Build history of the part. All positions in model axes, mm. Face numbers are marked on the shaded views. A direction names the side the tool comes from. Round coordinates to 2 decimals unless told otherwise and drop trailing zeros. Write each loop counter-clockwise with the first axis right and the second up, starting at its lowest first coordinate (ties: lowest second). Pieces come first, ordered by that corner, then holes. Notation, with made-up numbers: (60, 11.5) -> (96, 11.5) arc R22 cw to (96, 22.5) -> close; hole circle Ø10 at (4, 26). An arc over 180 degrees is marked (long way). Return JSON: item names as keys, results as strings.
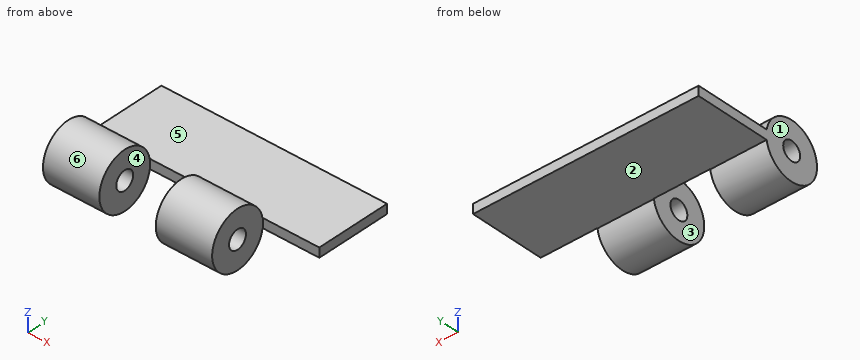
from build123d import *

# Parameters (mm, degrees)
F1_DEPTH = 1.5875
F2_W     = 19.05
F2_H     = 6.35


with BuildPart() as f1:
    # F0 (on Top) → F1 (new body, symmetric)
    with BuildSketch(Plane.XY):
        Polygon((76.2, 31.75), (0, 31.75), (0, 0), (19.05, 0), (19.05, 6.35), (38.1, 6.35), (38.1, 0), (57.15, 0), (57.15, 6.35), (76.2, 6.35), align=None)
    extrude(amount=F1_DEPTH, both=True)

    # F2 (on Top) → F3 (revolve)
    with BuildSketch(Plane.XY):
        with Locations((47.625, 3.175)):
            Rectangle(F2_W, F2_H)
        with Locations((9.525, 3.175)):
            Rectangle(F2_W, F2_H)
    revolve(axis=Axis((45.199081, -3.175, 0), (1, 0, 0)))


solid = f1.part
Q1. Saw through at A-A on z = 0. List the corners of the cut face in (x, y).
Verdict:
{"outline": "(0, -12.7) -> (19.05, -12.7) -> (19.05, -6.35) -> (0, -6.35) -> close; (0, 0) -> (19.05, 0) -> (19.05, 6.35) -> (38.1, 6.35) -> (38.1, 0) -> (57.15, 0) -> (57.15, 6.35) -> (76.2, 6.35) -> (76.2, 31.75) -> (0, 31.75) -> close; (38.1, -12.7) -> (57.15, -12.7) -> (57.15, -6.35) -> (38.1, -6.35) -> close"}
Q2. Wall check: L1, parallel to Z at x = 10.5, y = 19.5; L2, parallel to Y at x = 53.5, z = 0.5; L3, parallel to Y at x = 44.5, z = -1.5. Give the ranges that are in metal, low to high.
Verdict:
{"L1": "z = -1.59 to 1.59", "L2": "y = -12.69 to -6.31, -0.04 to 31.75", "L3": "y = -12.58 to -5.97, -0.38 to 31.75"}
Q3. Pin check, flat tips, straight feed: pin 1 Ø2 at (x, y) = (65.5, 7.5) entering from -Z; pin 2 Ø5 at (x, y) = (40, 22) entering from +Z; pin 3 Ø9.5 at (y, z) = (-4, -3) entering from +X; pin 4 Ø10 at (x, z) = (64.5, 7) entering from -Y. Stop position of each tip, or through.
Verdict:
{"pin 1": "stops at z = -1.59", "pin 2": "stops at z = 1.59", "pin 3": "stops at x = 57.15", "pin 4": "passes through"}
Q4. 3-axis set-ups, long thin cutter, end or side, ignore diameter. For the marked faces 5 and 6: which of +Z, -Z, +X, -X, +Y, -Y reach the whole face in a straight line?
Verdict:
{"face 5": "+Z, +X, -X, +Y", "face 6": "+X, -X"}
Q5. Saw through at D-D on x = 28.5. List the corners of the cut face in (y, z).
Verdict:
{"outline": "(6.35, -1.59) -> (31.75, -1.59) -> (31.75, 1.59) -> (6.35, 1.59) -> close"}
Q6. Saw through at C-C on z = -7.25. List the corners of the cut face in (x, y), then the cut area to 3 significant figures.
Verdict:
{"outline": "(0, -9.35) -> (19.05, -9.35) -> (19.05, 3) -> (0, 3) -> close; (38.1, -9.35) -> (57.15, -9.35) -> (57.15, 3) -> (38.1, 3) -> close", "area": "471 mm²"}
Q7. Two-plate mould, pull along X, no slides. Class the marked faces 1, 2, 3 and 4: +X half, -X half, draft (parallel to the pull), parting line (faces both ways), or undercut.
Verdict:
{"face 1": "-X half", "face 2": "draft", "face 3": "undercut", "face 4": "undercut"}
